Read the model definition and answer for the solid it produces. Units are mm, in the model's axes. Coordinates: 2 decimals unless noted, no trailing zeros. Loops run counter-clockwise (first coordinate to the right, second up) from the corner with the lowest first, then second, coordinate; pieces in that order, holes last. Notation, with made-up numbers: M 61,-1 L 92,-1 A25 ccw 92,22 Z; hole C 54.5,41 d10. An arc over 180 degrees is marked long. Put each result on its own line as item: value.
Autodesk Inventor part; units mm, degrees
ref_plane "Start plane" through (0, 0, -15.2763) normal (0, 0, 1) x (1, 0, 0)
ref_plane "End plane" through (0, 0, 37.7171) normal (0, 0, 1) x (1, 0, 0)
ref_plane "Work Plane4" through (0, 1.3151, 33.2269) normal (0, 0.7071, 0.7071) x (1, 0, 0)
ref_plane "Start plane" through (0, 0, -15.2763) normal (0, 0, 1) x (1, 0, 0)
ref_plane "End plane" through (0, 0, 37.7171) normal (0, 0, 1) x (1, 0, 0)
sketch "Sketch" plane through (0, 0, 0) normal (0, 0, 1) x (1, 0, 0)
  line L0 (12.7, -3.175) -> (-12.7, -3.175)
  line L1 (-12.7, -3.175) -> (-12.7, 3.175)
  line L2 (-12.7, 3.175) -> (12.7, 3.175)
  line L3 (12.7, 3.175) -> (12.7, -3.175)
  line L4 (-6, 0) -> (8, 0) construction
  line L5 (0, -30) -> (0, 40) construction
  line L6 (0, 54) -> (0, -44) construction
  line L7 (-17.78, 0) -> (17.78, 0) construction
  dimension "d0" = 6.35
  dimension "d1" = 25.4
  dimension "d4" = 12.7
  dimension "d5" = 3.175
extrude "Body" add sketch "Sketch" along normal up to surface (52.9934 mm away) from surface at -15.2763
sketch "Sketch3" plane through (0, 0, 0) normal (0, 0, 1) x (1, 0, 0)
  line L0 (0, 0) -> (10, 0)
ref_plane "Work Plane3" through (0, 0, 0) normal (0, -1, 0) x (1, 0, 0)
sketch "Sketch4" plane through (0, 0, 0) normal (0, -1, 0) x (1, 0, 0)
  line L0 (-2, -15.2763) -> (12, -15.2763)
  line L1 (-2, 37.7171) -> (12, 37.7171)
  dimension "d9" = 52.9934
ref_plane "Work Plane4" through (0, 1.3151, 33.2269) normal (0, 0.7071, 0.7071) x (1, 0, 0)
split "Split1" plane through (0, 1.3151, 33.2269) removes the side toward (0, 0.7071, 0.7071)
ref_plane "Work Plane5" through (0, -97.9118, -110.0131) normal (0, 0.7071, -0.7071) x (1, 0, 0)
split "Split2" plane through (0, -97.9118, -110.0131) removes the side toward (0, 0.7071, -0.7071)
equation "\"d0\" = G_W"
equation "\"d1\" = G_H"
equation "\"d4\" = 0.5 * d1"
equation "\"d5\" = 0.5 * d0"
equation "\"d2\" = G_L"
equation "\"G_W\" = 6.35"
equation "\"G_H\" = 25.4"
equation "\"G_L\" = d9"
equation "\"G_OFFSET_START\" = 15.27633"
equation "\"G_OFFSET_END\" = 8.98026"
equation "\"d6\" = -G_OFFSET_START"
equation "\"d7\" = G_OFFSET_END + B_L"
equation "\"B_L\" = 28.73682"
properties part number "AISC - 1/4x1 - 2.086" material "Steel, Mild"
1) Find section A-A, the plane x = 6.75. Write down the section's boundary in (y, z) (3 decimals).
Answer list:
outline: M -3.175,-15.276 L 3.175,-8.926 L 3.175,31.367 L -3.175,37.717 Z
2) Find section B-B, the plane y = -2.5. Write down the section's boundary in (x, z).
Answer list:
outline: M -12.7,-14.6 L 12.7,-14.6 L 12.7,37.04 L -12.7,37.04 Z
3) Given pin 1 Ø3 at (x, y) = (7.5, -1.5) entering from +Z, flat-ended and moving along its own axis, determine where the tip first touches the part or whether it passes through.
Answer list:
pin 1: stops at z = 37.54
4) Straight lines are drawn through the part: line 1 (Y direction, x = 3.75, z = 34) (3 decimals); line 2 (Z direction, x = -3, y = 2); line 3 (Z direction, x = 1, y = 0.25). For each, find the intervals that lie inside material, in ascending order. Write a range as [from, to].
Answer list:
line 1: y = [-3.175, 0.542]
line 2: z = [-10.1, 32.54]
line 3: z = [-11.85, 34.29]
